```python
from build123d import *

# Parameters (mm, degrees)
SKETCH_1_W          = 40
SKETCH_1_H          = 30
EXTRUDE_1_DEPTH     = 4
SKETCH_2_W          = 22.2
SKETCH_2_H          = 10.2
CUT_EXTRUDE_1_DEPTH = 10
SKETCH_3_W          = 10.2
SKETCH_3_H          = 4
EXTRUDE_2_DEPTH     = 5


with BuildPart() as part:
    # 草圖1 → 填料-伸長1 (new body)
    with BuildSketch(Plane(origin=(0, 0, 0), x_dir=(1, 0, 0), z_dir=(0, 1, 0))):
        with Locations((20, 15)):
            Rectangle(SKETCH_1_W, SKETCH_1_H)
    extrude(amount=EXTRUDE_1_DEPTH)

    # 草圖2 → 除料-伸長1 (cut)
    with BuildSketch(Plane(origin=(0, 4, 0), x_dir=(1, 0, 0), z_dir=(0, 1, 0))):
        with Locations((28.9, 15)):
            Rectangle(SKETCH_2_W, SKETCH_2_H)
    extrude(amount=-CUT_EXTRUDE_1_DEPTH, mode=Mode.SUBTRACT)

    # 草圖3 → 填料-伸長2 (add)
    with BuildSketch(Plane(origin=(17.8, 0, 0), x_dir=(0, 0, -1), z_dir=(1, 0, 0))):
        with Locations((15, 2)):
            Rectangle(SKETCH_3_W, SKETCH_3_H)
    extrude(amount=EXTRUDE_2_DEPTH)


solid = part.part
```
Part model, mm, in its own coordinate system. A direction names the side the tool comes from. Round coordinates to 2 decimals unless told otherwise and drop trailing zeros. Order: outer loops, then holes, each group sorted by start corner. A loop starts at its lowest first (then second) coordinate and runs counter-clockwise, first axis right, second up. Notation, with made-up numbers: M 47.5,19 L 83.5,19 A26 ccw 83.5,57 Z; hole C 49.25,-38.5 d9. An arc over 180 degrees is marked long. Answer in a Markdown table with one row per item. Add a question column.
Q1. Pin check, flat tip, straight feed: pin 1 (1 mm diameter, centred on y = 3, z = -11.5, fed in from +X). Stop position of the tip, or through.
Q2. Mould opens along Z. For faces 3 (the face through (31, 2, -20.1)), 4 (the face through (20, 2, 0)), 5 (the face through (0, 2, -15)), 6 (the face through (20, 2, -30)) say: +Z half, -Z half, draft (parallel to the pull), parting line (faces both ways), or undercut.
Q3. Cut at A-A on x = 27. Give the cut face in (y, z).
Q4. Cut at B-B on y = 1.4. Give the cut face in (x, z), and give its area (3 significant figures).
Q5. 3-axis set-ups, long thin cutter, end or side, ignore diameter. For faces 1 (the face through (31, 2, -9.9)), 2 (the face through (40, 2, -25)): which of +Z, -Z, +X, -X, +Y, -Y reach the whole face in a straight line?
Q6. Wall check: L1, parallel to Z at x = 28, y = 3.65; L2, parallel to X at y = 2.25, z = -18. Give the ranges that are in metal, low to high. Write a range as from..to.
Q7. Cut at C-C on z = -11.75. Give the cut face in (x, y).
Established:
| question | item | result |
|---|---|---|
| 1 | pin 1 | stops at x = 22.8 |
| 2 | face 3 | undercut |
| 2 | face 4 | +Z half |
| 2 | face 5 | draft |
| 2 | face 6 | -Z half |
| 3 | outline | M 0,-30 L 4,-30 L 4,-20.1 L 0,-20.1 Z; M 0,-9.9 L 4,-9.9 L 4,0 L 0,0 Z |
| 4 | outline | M 0,-30 L 40,-30 L 40,-20.1 L 22.8,-20.1 L 22.8,-9.9 L 40,-9.9 L 40,0 L 0,0 Z |
| 4 | area | 1,020 mm2 |
| 5 | face 1 | +X, +Y, -Y |
| 5 | face 2 | +Z, -Z, +X, +Y, -Y |
| 6 | L1 | z = -30..-20.1, -9.9..0 |
| 6 | L2 | x = 0..22.8 |
| 7 | outline | M 0,0 L 22.8,0 L 22.8,4 L 0,4 Z |
